```python
from build123d import *

# Parameters (mm, degrees)
F1_DEPTH = 70
F2_W     = 20
F2_H     = 30
F3_DEPTH = 70.001
F4_W     = 40
F4_H     = 20
F5_DEPTH = 130.001


with BuildPart() as f1:
    # F0 (on Front) → F1 (new body)
    with BuildSketch(Plane.XZ):
        Polygon((65, -35), (65, 35), (15, 35), (-25, -5), (-65, -5), (-65, -35), (-25, -35), align=None)
    extrude(amount=F1_DEPTH)

    # F2 (on face) → F3 (cut, through all)
    with BuildSketch(Plane(origin=(0, 0, -35), x_dir=(1, 0, 0), z_dir=(0, 0, -1))):
        with Locations((-55, 35)):
            Rectangle(F2_W, F2_H)
    extrude(amount=-F3_DEPTH, mode=Mode.SUBTRACT)

    # F4 (on face) → F5 (cut, through all)
    with BuildSketch(Plane.YZ.offset(65)):
        with Locations((-35, 15)):
            Rectangle(F4_W, F4_H)
    extrude(amount=-F5_DEPTH, mode=Mode.SUBTRACT)


solid = f1.part
```
Verification items for the finished model (mm, model axes). A direction names the side the tool comes from. Coordinates: 2 decimals unless noted, no trailing zeros. Loops run counter-clockwise (first coordinate to the right, second up) from the corner with the lowest first, then second, coordinate; pieces in that order, holes last. Notation, with made-up numbers: (74.5, 82) - (107.5, 82) arc R16 ccw to (107.5, 112) - close; hole circle Ø9 at (83.25, 45). An arc over 180 degrees is marked (long way). Put each result on its own line as item: value.
Item 1: Gauge pin test, flat ends, axial feed: pin 1 Ø15 at (y, z) = (-34.5, -22.5) entering from -X; pin 2 Ø3 at (x, y) = (-48.5, -8.5) entering from +Z; pin 3 Ø12 at (y, z) = (-37, 9.5) entering from -X. Record the tip position at first contact, or that the pin passes through.
Conclusion:
pin 1: stops at x = -45
pin 2: stops at z = -5
pin 3: stops at x = -16.5
Item 2: Section check C-C (x = 12). Enter the section's corners in (y, z), then the cut area to 3 significant figures.
Conclusion:
outline: (-70, -35) - (0, -35) - (0, 32) - (-70, 32) - close; hole (-55, 5) - (-15, 5) - (-15, 25) - (-55, 25) - close
area: 3,890 mm2
Item 3: Section check B-B (y = -31). Enter the section's corners in (x, z), then the cut area to 3 significant figures.
Conclusion:
outline: (-45, -35) - (65, -35) - (65, 5) - (-15, 5) - (-25, -5) - (-45, -5) - close; (5, 25) - (65, 25) - (65, 35) - (15, 35) - close
area: 4,700 mm2
Item 4: Section check A-A (z = 23.5). Enter the section's corners in (x, y), then the cut area to 4 significant figures.
Conclusion:
outline: (3.5, -70) - (65, -70) - (65, -55) - (3.5, -55) - close; (3.5, -15) - (65, -15) - (65, 0) - (3.5, 0) - close
area: 1,845 mm2
Item 5: Draft check along Z on faces 1 (the face through (34, -15, 15)), 2 (the face through (-65, -60, -20)), 3 (the face through (9, -35, 29)), 4 (the face through (-1, -35, -35)). Enter one of: pulls with the +Z half, pulls with the -Z half, needs draft (parallel to the pull), parting line crosses it, or undercut.
Conclusion:
face 1: undercut
face 2: needs draft
face 3: pulls with the +Z half
face 4: pulls with the -Z half
Item 6: Scan lines: line 1 along Z through (x, y) = (17.5, -52.5); line 2 along Y through (x, z) = (30.5, 14.5); line 3 along X through (y, z) = (-39, -21). Record each from-to range of solid material in increasing order.
Conclusion:
line 1: z = -35 to 5, 25 to 35
line 2: y = -70 to -55, -15 to 0
line 3: x = -45 to 65
Item 7: Section check D-D (z = -15). Enter the section's corners in (x, y).
Conclusion:
outline: (-65, -70) - (65, -70) - (65, 0) - (-65, 0) - (-65, -20) - (-45, -20) - (-45, -50) - (-65, -50) - close
Item 8: Set-up check for faces 5 (the face through (-44.7, -34.5, -5)), 6 (the face through (40, -35, 35)), 7 (the face through (14, 0, -7)), 8 (the face through (-55, -20, -20)), 9 (the face through (35, -35, 25)): record each of +Z, -Z, +X, -X, +Y, -Y from which the full face is reachable in a straight line by a thin tool's end or side.
Conclusion:
face 5: +Z, -X, +Y, -Y
face 6: +Z, +X, -X, +Y, -Y
face 7: +Z, -Z, +X, -X, +Y
face 8: +Z, -Z, -X
face 9: +X, -X
